The model under review builds one solid part; all positions refer to its coordinate system, in mm. Face numbers are marked on the shaded views. Round coordinates to 2 decimals unless told otherwise and drop trailing zeros. Order: outer loops, then holes, each group sorted by start corner. A loop starts at its lowest first (then second) coordinate and runs counter-clockwise, first axis right, second up. Notation, with made-up numbers: M -16,-21 L 25,-21 A26 cw 25,-3 Z; hole C 20.25,42 d9. An arc over 180 degrees is marked long. Answer as a JSON object with one key per item and string values. Group by question number.
1) Insertion check: pin 1 Ø1 at (y, z) = (-0.5, -3.5) entering from -X; pin 2 Ø2 at (y, z) = (1, -0.5) entering from +X. Each pin has a flat end and moves straight along its axis. Give the tip position at first contact, or say it passes through.
2) The part is to be moulded in two halves that separate along Y. For the marked faces 1, 2 and 3, say which applies: +Y half, -Y half, draft (parallel to the pull), parting line (faces both ways), or undercut.
3) Consider section A-A, the plane x = 0. Write out the cut boundary in (y, z), then the cut area to 3 significant figures.
4) Consider section D-D, the plane x = -1.8. Write out the cut boundary in (y, z).
5) To check wall thickness, follow line 1 (Y direction, x = 0, z = -3); line 2 (X direction, y = -0.15, z = -3); line 3 (Z direction, x = 0.8, y = -1.85). State the ranges of each line that lie inside material, in increasing order.
6) Consider section C-C, the plane z = -2.25. Write out the cut boundary in (x, y).
```python
from build123d import *


with BuildPart() as part:
    # Esquisse1 → base (revolve)
    with BuildSketch(Plane(origin=(0, 0, 0), x_dir=(0, 0, -1), z_dir=(1, 0, 0)), mode=Mode.PRIVATE) as base_sk:
        with BuildLine():
            Line((6.2, 1), (6.2, 1.3))
            Line((6.2, 1.3), (0.1, 1.3))
            ThreePointArc((0.1, 1.3), (0.029289322, 1.329289322), (0, 1.4))
            Line((0, 1.4), (0, 2.1))
            Line((0, 2.1), (-0.3, 2.1))
            Line((-0.3, 2.1), (-0.3, 1.4))
            ThreePointArc((-0.3, 1.4), (-0.182842712, 1.117157288), (0.1, 1))
            Line((0.1, 1), (6.2, 1))
        make_face()
    revolve(base_sk.sketch.rotate(Axis((0, 0, 0.3), (0, 0, -1)), 90), axis=Axis((0, 0, 0.3), (0, 0, -1)))


solid = part.part
```
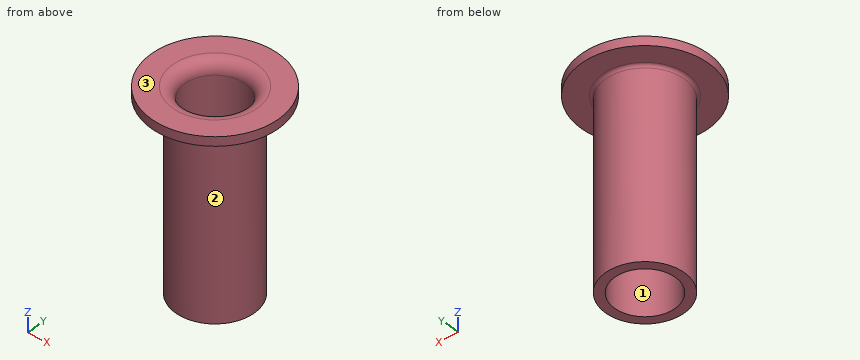
Results list:
{
 "1": {"pin 1": "x = -1.3", "pin 2": "x = 2.1"},
 "2": {"face 1": "undercut", "face 2": "parting line", "face 3": "draft"},
 "3": {"outline": "M -2.1,0 L -1.4,0 A0.1 cw -1.3,-0.1 L -1.3,-6.2 L -1,-6.2 L -1,-0.1 A0.4 ccw -1.4,0.3 L -2.1,0.3 Z; M 1,-6.2 L 1.3,-6.2 L 1.3,-0.1 A0.1 cw 1.4,0 L 2.1,0 L 2.1,0.3 L 1.4,0.3 A0.4 ccw 1,-0.1 Z", "area": "4.32 mm^2"},
 "4": {"outline": "M -1.08,0 L 1.08,0 L 1.08,0.3 L -1.08,0.3 Z"},
 "5": {"line 1": "-1.3 to -1, 1 to 1.3", "line 2": "-1.29 to -0.99, 0.99 to 1.29", "line 3": "0 to 0.3"},
 "6": {"outline": "C 0,0 d2.6; hole C 0,0 d2"}
}
